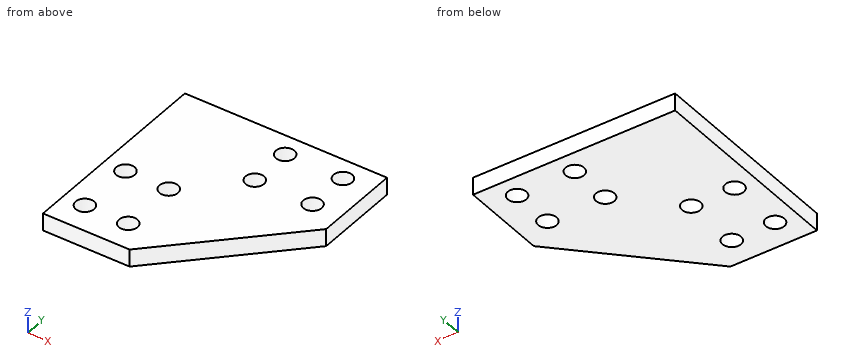
```python
from build123d import *

# Parameters (mm, degrees)
SKETCH_1_R      = 1.6
EXTRUDE_1_DEPTH = 3


with BuildPart() as part:
    # 草图1 → 凸台-拉伸1 (new body)
    with BuildSketch(Plane.XY):
        Polygon((0, 0), (35, 0), (35, -15), (15, -35), (0, -35), align=None)
        with Locations((3.75, -30)):
            Circle(SKETCH_1_R, mode=Mode.SUBTRACT)
        with Locations(Location((11.25, -30, 0), (0, 0, 180))):
            Circle(SKETCH_1_R, mode=Mode.SUBTRACT)
        with Locations((11.25, -20)):
            Circle(SKETCH_1_R, mode=Mode.SUBTRACT)
        with Locations(Location((3.75, -20, 0), (0, 0, 180))):
            Circle(SKETCH_1_R, mode=Mode.SUBTRACT)
        with Locations((30, -3.75)):
            Circle(SKETCH_1_R, mode=Mode.SUBTRACT)
        with Locations(Location((30, -11.25, 0), (0, 0, 180))):
            Circle(SKETCH_1_R, mode=Mode.SUBTRACT)
        with Locations((20, -11.25)):
            Circle(SKETCH_1_R, mode=Mode.SUBTRACT)
        with Locations(Location((20, -3.75, 0), (0, 0, 180))):
            Circle(SKETCH_1_R, mode=Mode.SUBTRACT)
    extrude(amount=EXTRUDE_1_DEPTH)


solid = part.part
```
The listing builds one solid part. Answer for the finished solid, in the listing's coordinates (mm). Give positions to 0.01 mm unless a question says otherwise; leave off trailing zeros. Write each loop counter-clockwise with the first axis right and the second up, starting at its lowest first coordinate (ties: lowest second). Pieces come first, ordered by that corner, then holes. Notation, with made-up numbers: (89.25, 46.25) - (115.25, 46.25) arc R25 ccw to (115.25, 65.25) - close; hole circle Ø4 at (-25.5, 63). An arc over 180 degrees is marked (long way). Use one line per item in the form item = value. Start each with the question number.
1) Find section B-B on z = 1.5. Count the separate pieces of the cut face and the enclosed holes in it, plus the area to 3 significant figures.
2) Find section D-D on x = 23. Determine the outline of the cut face in (y, z), plus the area to 3 significant figures.
3) Consider line 1 along Y through (x, z) = (11.25, 1.6); line 2 along Y through (x, z) = (30.5, 1); line 3 along X through (y, z) = (-4.5, 0.55). Determine where each line is inside the solid, lowest interval first. Write a range as from..to.
4) Find section A-A on y = -30. Determine the outline of the cut face in (x, z).
5) Find section C-C on x = 11.25. Determine the outline of the cut face in (y, z), plus the area to 3 significant figures.
Geometry results:
q1.separate_pieces = 1
q1.enclosed_holes = 8
q1.area = 961 mm2
q2.outline = (-27, 0) - (0, 0) - (0, 3) - (-27, 3) - close
q2.area = 81.0 mm2
q3.line_1 = -35..-31.6, -28.4..-21.6, -18.4..0
q3.line_2 = -19.5..-12.77, -9.73..-5.27, -2.23..0
q3.line_3 = 0..18.59, 21.41..28.59, 31.41..35
q4.outline = (0, 0) - (2.15, 0) - (2.15, 3) - (0, 3) - close; (5.35, 0) - (9.65, 0) - (9.65, 3) - (5.35, 3) - close; (12.85, 0) - (20, 0) - (20, 3) - (12.85, 3) - close
q5.outline = (-35, 0) - (-31.6, 0) - (-31.6, 3) - (-35, 3) - close; (-28.4, 0) - (-21.6, 0) - (-21.6, 3) - (-28.4, 3) - close; (-18.4, 0) - (0, 0) - (0, 3) - (-18.4, 3) - close
q5.area = 85.8 mm2
